Verification items for the finished model (mm, model axes). A direction names the side the tool comes from. Round coordinates to 2 decimals unless told otherwise and drop trailing zeros. Write each loop counter-clockwise with the first axis right and the second up, starting at its lowest first coordinate (ties: lowest second). Pieces come first, ordered by that corner, then holes. Notation, with made-up numbers: (2.5, -16) - (60.5, -16) arc R22 cw to (60.5, -5) - close; hole circle Ø5 at (58, 82.5). An arc over 180 degrees is marked (long way). Answer as a JSON object with one key per item and string values. Group by question number.
1) Set-up check for faces 4 (the flat face through (41, 0, -8)), 5 (the cylindrical face through (43.995, -10.088, -6.591)), 6 (the flat face through (-27.5, -24, -1)), 7 (the flat face through (-6, -12, -7)): record each of +Z, -Z, +X, -X, +Y, -Y from which the full face is reachable in a straight line by a thin tool's end or side.
2) Section check A-A (y = -11). Enter the section's corners in (x, z), then the cut area to 3 significant figures.
3) Section check D-D (z = -9.25). Enter the section's corners in (x, y).
4) Thickness scan on line 1 (Y direction, x = -43, z = -4.5); line 2 (Z direction, x = -5, y = -11.5); line 3 (Y direction, x = 28, z = -4.5). Record the ranges inside material, lowest first.
5) Go/stop test with flat-tipped pins: pin 1 Ø3 at (x, z) = (34, -9) entering from -Y; pin 2 Ø3.5 at (x, y) = (-43, -11) entering from -Z; pin 3 Ø5 at (x, y) = (-26.5, -28) entering from -Z; pin 4 Ø2 at (x, y) = (-43, 11) entering from -Z. Record where each tip stops, or that it passes through.
6) Mould release check, pull along Z, two halves, no side actions. Record for faces 1 (the flat face through (1, 15, -7)), 2 (the flat face through (0, -12, -10.5)), 3 (the flat face through (1, 10, -13)): +Z half, -Z half, draft (parallel to the pull), parting line (faces both ways), or undercut.
7) Section check C-C (x = 20). Enter the section's corners in (y, z).
8) Section check B-B (y = 11). Enter the section's corners in (x, z).
```python
from build123d import *

# Parameters (mm, degrees)
SKETCH001_W          = 94
SKETCH001_H          = 30
PAD_DEPTH            = 13
SKETCH002_R          = 1.35
HOLE_DEPTH           = 25
SKETCH_W             = 82
SKETCH_H             = 18
POCKET_DEPTH         = 10
SKETCH003_W          = 55
SKETCH003_H          = 21
PAD001_DEPTH         = 3
FILLET_R             = 1
SKETCH004_R          = 3
HOLE001_DEPTH        = 25
SKETCH010_W          = 12
SKETCH010_H          = 7.5
POCKET001_DEPTH      = 6
BODY_PLACEMENT_ANGLE = 180


with BuildPart() as part:
    # Sketch001 → Pad (new body)
    with BuildSketch(Plane.XY):
        Rectangle(SKETCH001_W, SKETCH001_H)
    extrude(amount=-PAD_DEPTH)

    # Sketch002 (on Face5 of Pad) → Hole (cut)
    with BuildSketch(Plane.XY):
        with Locations((-43, 11)):
            Circle(SKETCH002_R)
        with Locations((-43, -11)):
            Circle(SKETCH002_R)
        with Locations((43, 11)):
            Circle(SKETCH002_R)
        with Locations((43, -11)):
            Circle(SKETCH002_R)
    extrude(amount=-HOLE_DEPTH, mode=Mode.SUBTRACT)

    # Sketch → Pocket (cut)
    with BuildSketch(Plane.XY):
        Rectangle(SKETCH_W, SKETCH_H)
    extrude(amount=-POCKET_DEPTH, mode=Mode.SUBTRACT)

    # Sketch003 (on Face5 of Pocket) → Pad001 (join)
    with BuildSketch(Plane(origin=(0, 0, -13), x_dir=(1, 0, 0), z_dir=(0, 0, -1))):
        with Locations((0, 22.5)):
            Rectangle(SKETCH003_W, SKETCH003_H)
    extrude(amount=-PAD001_DEPTH)

    # Fillet
    fillet_edges = [part.edges().sort_by_distance(p)[0] for p in [
        (47, -15, -6.5),
        (47, 15, -6.5),
        (-47, 15, -6.5),
        (-47, -15, -6.5),
    ]]
    fillet(fillet_edges, radius=FILLET_R)

    # Sketch004 (on Face22 of Fillet) → Hole001 (cut)
    with BuildSketch(Plane.XY.offset(-10)):
        with Locations((20, -23)):
            Circle(SKETCH004_R)
        with Locations((-20, -23)):
            Circle(SKETCH004_R)
    extrude(amount=-HOLE001_DEPTH, mode=Mode.SUBTRACT)

    # Sketch010 (on Face7 of Hole001) → Pocket001 (cut)
    with BuildSketch(Plane.XZ.offset(15)):
        with Locations((0, -6.25)):
            Rectangle(SKETCH010_W, SKETCH010_H)
    extrude(amount=-POCKET001_DEPTH, mode=Mode.SUBTRACT)


with BuildPart() as part_1:
    # Body placement: moved
    add(part.part.moved(Location((0, 0, -13))).rotate(Axis((0, 0, -13), (0, 1, 0)), BODY_PLACEMENT_ANGLE))


solid = part_1.part
```
Returned:
{
 "1": {"face 4": "-Z", "face 5": "+Z, -Z", "face 6": "+Z, -Z, -X, -Y", "face 7": "-Y"},
 "2": {"outline": "(-47, -13) - (-44.35, -13) - (-44.35, 0) - (-47, 0) - close; (-41.65, -13) - (41.65, -13) - (41.65, 0) - (-41.65, 0) - close; (44.35, -13) - (47, -13) - (47, 0) - (44.35, 0) - close; hole (-6, -10.5) - (6, -10.5) - (6, -3) - (-6, -3) - close", "area": "1,060 mm2"},
 "3": {"outline": "(-47, -14) arc R1 ccw to (-46, -15) - (-6, -15) - (-6, -9) - (-41, -9) - (-41, 9) - (41, 9) - (41, -9) - (6, -9) - (6, -15) - (46, -15) arc R1 ccw to (47, -14) - (47, 14) arc R1 ccw to (46, 15) - (-46, 15) arc R1 ccw to (-47, 14) - close; hole circle Ø2.7 at (-43, -11); hole circle Ø2.7 at (-43, 11); hole circle Ø2.7 at (43, -11); hole circle Ø2.7 at (43, 11)"},
 "4": {"line 1": "-15 to -12.35, -9.65 to 9.65, 12.35 to 15", "line 2": "-13 to -10.5, -3 to 0", "line 3": "-15 to -9, 9 to 15"},
 "5": {"pin 1": "y = -15", "pin 2": "z = -13", "pin 3": "z = -3", "pin 4": "through"},
 "6": {"face 1": "draft", "face 2": "undercut", "face 3": "-Z half"},
 "7": {"outline": "(-33, -3) - (-26, -3) - (-26, 0) - (-33, 0) - close; (-20, -3) - (-15, -3) - (-15, -13) - (-9, -13) - (-9, -3) - (9, -3) - (9, -13) - (15, -13) - (15, 0) - (-20, 0) - close"},
 "8": {"outline": "(-47, -13) - (-44.35, -13) - (-44.35, 0) - (-47, 0) - close; (-41.65, -13) - (41.65, -13) - (41.65, 0) - (-41.65, 0) - close; (44.35, -13) - (47, -13) - (47, 0) - (44.35, 0) - close"}
}
